Geometry: final body of the model. Coordinates: model frame, mm. Face numbers are marked on the shaded views. A direction names the side the tool comes from. Give positions to 0.01 mm unless a question says otherwise; leave off trailing zeros. Loops run counter-clockwise (first coordinate to the right, second up) from the corner with the lowest first, then second, coordinate; pieces in that order, holes last. Notation, with made-up numbers: M 30,-33 L 40,-33 A21 ccw 40,3 Z; hole C 32,-5 d7. An arc over 180 degrees is marked long. One line per question, with ' | ' between items. Start each with the question number.
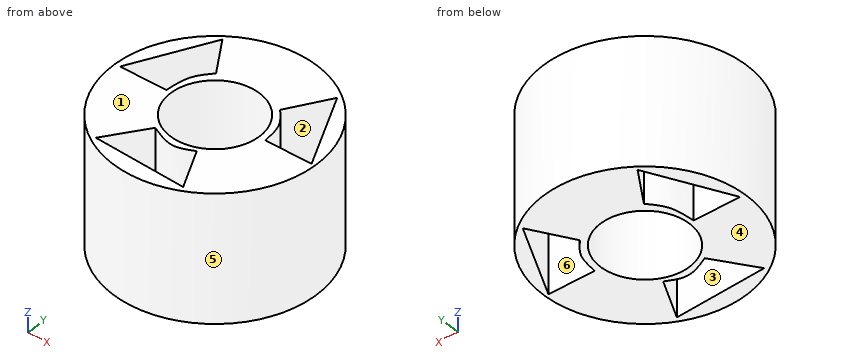
from build123d import *

# Parameters (mm, degrees)
F0_R     = 4
F1_DEPTH = 2.5
F2_R     = 1.75
F3_DEPTH = 11.3
F6_DEPTH = 8.5


with BuildPart() as f1:
    # F0 (on Top) → F1 (new body, symmetric)
    with BuildSketch(Plane.XY):
        Circle(F0_R)
    extrude(amount=F1_DEPTH, both=True)

    # F2 (on face) → F3 (cut)
    with BuildSketch(Plane.XY.offset(2.5)):
        Circle(F2_R)
    extrude(amount=-F3_DEPTH, mode=Mode.SUBTRACT)

    # F5 (on face) → F6 (cut)
    with BuildSketch(Plane.XY.offset(2.5)):
        with BuildLine():
            add(Edge.make_bspline(
                [(2.0119966939, 0), (1.9826024943, 0.2954333995), (1.924894753, 0.8754387886), (1.5462774399, 1.2772605749), (1.360513852, 1.4744091313)],
                knots=[0, 0, 0, 0, 0.5093631973, 1, 1, 1, 1], degree=3))
            Line((2.0119966939, 0), (3.8635805249, 0))
            Line((3.8635805249, 0), (2.3034499027, 3.0688282568))
            Line((2.3034499027, 3.0688282568), (1.360513852, 1.4744091313))
        make_face()
        with BuildLine():
            Line((-3.7999181077, 0), (-2.1026332397, 0))
            Line((-2.1026332397, 0), (-1.9483346259, 0))
            add(Edge.make_bspline(
                [(-1.3311400544, 1.6287077451), (-1.5110569531, 1.4224997977), (-1.8877122283, 0.9908043222), (-1.9275343397, 0.3399570839), (-1.9483346259, 0)],
                knots=[0, 0, 0, 0, 0.4776699295, 1, 1, 1, 1], degree=3))
            Line((-1.3311400544, 1.6287077451), (-2.2912204731, 3.0688282568))
            Line((-2.2912204731, 3.0688282568), (-3.7999181077, 0))
        make_face()
        with BuildLine():
            Line((-0.9711100138, -1.6801406164), (-2.0340562332, -3.2402712386))
            Line((-2.0340562332, -3.2402712386), (1.6176782083, -3.428858472))
            Line((1.6176782083, -3.428858472), (0.7604635903, -1.7658622237))
            add(Edge.make_bspline(
                [(-0.9711100138, -1.6801406164), (-0.637698637, -1.848903582), (-0.0099582222, -2.1666471906), (0.514541214, -1.8937947275), (0.7604635903, -1.7658622237)],
                knots=[0, 0, 0, 0, 0.5311293792, 1, 1, 1, 1], degree=3))
        make_face()
    extrude(amount=-F6_DEPTH, mode=Mode.SUBTRACT)


solid = f1.part
Q1. Section B-B, the plane z = -0.4. Count the separate pieces of the cut face and the enclosed holes in it, plus the area to 3 significant figures.
Q2. Section A-A, the plane x = -3.25. Output: boundary loops of the cut face in (y, z), plus the area to 3 significant figures.
Q3. Set-up query: the marked faces 1 and 2. Return all of +Z, -Z, +X, -X, +Y, -Y with unobstructed straight access to the full face (end or side cutting, diameter ignored); none if empty.
Q4. Contact query for flat-ended pins moving along their axis: pin 1 (0.9 mm diameter, centred on x = 3, z = -0.5, fed in from +Y); pin 2 (0.6 mm diameter, centred on x = -3, z = 1, fed in from +Y). Output: stop coordinate, or through.
Q5. Draft query along Y for the marked faces 3, 4, 5 and 6. Return one class per face: released by +Y, released by -Y, zero draft, split by the parting line, or undercut.
Q6. Material intervals for L1, parallel to Y at x = 0, z = -0.45; L2, parallel to Y at x = -1.25, z = 0.6; L3, parallel to X at y = 2.75, z = -2.3, sorted ascending.
Model answer:
1) separate pieces: 1 | enclosed holes: 4 | area: 28.9 mm^2
2) outline: M -2.33,-2.5 L 0,-2.5 L 0,2.5 L -2.33,2.5 Z; M 1.12,-2.5 L 2.33,-2.5 L 2.33,2.5 L 1.12,2.5 Z | area: 17.7 mm^2
3) face 1: +Z, +X, -X, +Y, -Y | face 2: +Z, -Z
4) pin 1: stops at y = 3.08 | pin 2: stops at y = 2.95
5) face 3: undercut | face 4: zero draft | face 5: split by the parting line | face 6: undercut
6) L1: y = -4 to -3.35, -2.02 to -1.75, 1.75 to 4 | L2: y = -3.8 to -3.28, -2.09 to -1.22, 1.22 to 3.8 | L3: x = -2.9 to -2.45, -2.08 to 2.11, 2.47 to 2.9
